Model file for the job. Use its own axes, mm. Give positions to 0.01 mm unless a question says otherwise; leave off trailing zeros. Loops run counter-clockwise (first coordinate to the right, second up) from the corner with the lowest first, then second, coordinate; pieces in that order, holes last. Notation, with made-up numbers: M -34.75,88.25 L 11.25,88.25 A33 cw 11.25,127.25 Z; hole C 10,83 d6. An arc over 180 degrees is marked long. Answer in a Markdown table with one row per item.
```python
from build123d import *

# Parameters (mm, degrees)
SKETCH_1_W            = 15
SKETCH_1_H            = 70
EXTRUDE_1_DEPTH       = 2
HOLE_WIZARD_M41_D     = 3.3
HOLE_WIZARD_M41_DEPTH = 11.5
HOLE_WIZARD_M41_TIP   = 0.991420021
FILLET_1_R            = 2


with BuildPart() as part:
    # Эскиз1 → Бобышка-Вытянуть1 (new body)
    with BuildSketch(Plane.XY):
        Rectangle(SKETCH_1_W, SKETCH_1_H)
    extrude(amount=EXTRUDE_1_DEPTH)

    # Отверстие обработанное метчиком M41
    with Locations(Plane.XY.offset(2)):
        with Locations((0, 25), (0, -25), (0, -10), (0, 10)):
            Hole(HOLE_WIZARD_M41_D / 2, depth=HOLE_WIZARD_M41_DEPTH)
            with Locations((0, 0, -(HOLE_WIZARD_M41_DEPTH + HOLE_WIZARD_M41_TIP / 2))):  # 118° drill point
                Cone(0, HOLE_WIZARD_M41_D / 2, HOLE_WIZARD_M41_TIP, mode=Mode.SUBTRACT)

    # Скругление1
    fillet_1_edges = [part.edges().sort_by_distance(p)[0] for p in [
        (7.5, -35, 1),
        (-7.5, -35, 1),
        (-7.5, 35, 1),
        (7.5, 35, 1),
    ]]
    fillet(fillet_1_edges, radius=FILLET_1_R)


solid = part.part
```
Q1. Mould opens along X. For faces 1 (the face through (0.4, 8.4, 1)), 2 (the face through (6.9, -34.43, 1.01)), 3 (the face through (0, 0, 0)), 4 (the face through (0.215, 26.636, 0.986)) say: released by +X, released by -X, zero draft, split by the parting line, or undercut.
Reported:
| item | result |
|---|---|
| face 1 | undercut |
| face 2 | released by +X |
| face 3 | zero draft |
| face 4 | undercut |
Q2. Saw through at C-C (z = 1.7). Give the cut face in (x, y), and give its area (3 significant figures).
Reported:
| item | result |
|---|---|
| outline | M -7.5,-33 A2 ccw -5.5,-35 L 5.5,-35 A2 ccw 7.5,-33 L 7.5,33 A2 ccw 5.5,35 L -5.5,35 A2 ccw -7.5,33 Z; hole C 0,-25 d3.3; hole C 0,-10 d3.3; hole C 0,10 d3.3; hole C 0,25 d3.3 |
| area | 1,010 mm² |
Q3. Probe probe 1 along Y at (x, z) = (0, 0.95); probe 2 along Y at (x, z) = (-1.5, 0.35); probe 3 along X at (y, z) = (9, 1.6). List the from-to ranges inside material, lowest first.
Reported:
| item | result |
|---|---|
| probe 1 | -35 to -26.65, -23.35 to -11.65, -8.35 to 8.35, 11.65 to 23.35, 26.65 to 35 |
| probe 2 | -35 to -25.69, -24.31 to -10.69, -9.31 to 9.31, 10.69 to 24.31, 25.69 to 35 |
| probe 3 | -7.5 to -1.31, 1.31 to 7.5 |
Q4. Drop a flat-ended pin along its axis: pin 1 (3 mm diameter, centred on x = 0, y = -25, fed in from -Z). Give the stop position or say it passes through.
Reported:
| item | result |
|---|---|
| pin 1 | through |
Q5. Saw through at A-A (x = 0). Give the cut face in (y, z), and give its area (3 significant figures).
Reported:
| item | result |
|---|---|
| outline | M -35,0 L -26.65,0 L -26.65,2 L -35,2 Z; M -23.35,0 L -11.65,0 L -11.65,2 L -23.35,2 Z; M -8.35,0 L 8.35,0 L 8.35,2 L -8.35,2 Z; M 11.65,0 L 23.35,0 L 23.35,2 L 11.65,2 Z; M 26.65,0 L 35,0 L 35,2 L 26.65,2 Z |
| area | 114 mm² |
Q6. Saw through at B-B (y = 10). Give the cut face in (x, z), and give its area (3 significant figures).
Reported:
| item | result |
|---|---|
| outline | M -7.5,0 L -1.65,0 L -1.65,2 L -7.5,2 Z; M 1.65,0 L 7.5,0 L 7.5,2 L 1.65,2 Z |
| area | 23.4 mm² |
